Geometry check sheet. Reference: the model listing, model coordinates, mm. Round coordinates to 2 decimals unless told otherwise and drop trailing zeros. Order: outer loops, then holes, each group sorted by start corner. A loop starts at its lowest first (then second) coordinate and runs counter-clockwise, first axis right, second up.
(1) Sectioned sample at A-A (y = 2.25). Record the boundary of the cut face in (x, z), plus the area to 3 significant figures.
(2) Sectioned sample at B-B (x = 86.5). Record the boundary of the cut face in (y, z), plus the area to 3 significant figures.
(3) Material ranges on line 1 along Z through (x, y) = (93.5, 3); line 2 along X through (y, z) = (3.65, 127), recorded low to high.
Autodesk Fusion 360 part; units mm, degrees
sketch "Sketch1" plane through (0, 0, 0) normal (0, 1, 0) x (1, 0, 0)
  line L0 (0, 0) -> (170, 0)
  line L1 (170, 0) -> (170, -376)
  line L2 (170, -376) -> (0, -376)
  line L3 (0, -376) -> (0, 0)
  dimension "d1" = 170
  dimension "d2" = 376
extrude "Extrude1" add sketch "Sketch1" along normal blind 5
sketch "Sketch2" plane through (0, 0, 0) normal (-1, 0, 0) x (0, 0, 1)
  line L0 (0, 0) -> (376, 0)
  line L1 (376, 0) -> (376, 5)
  line L2 (376, 5) -> (0, 5)
  line L3 (0, 5) -> (0, 0)
extrude "Extrude2" cut 1 faces at (56.6667, 1.6667, 0) along direction (0, 0, 1) blind 3
extrude "Extrude3" cut 1 faces at (170, 1.6667, 127.3333) along direction (-1, 0, 0) blind 3
extrude "Extrude4" add 1 faces at (55.6667, 1.6667, 3) along direction (0, 0, -1) blind 3
extrude "Extrude5" add 1 faces at (167, 1.6667, 250.6667) along direction (1, 0, 0) blind 2
extrude "Extrude6" add 1 faces at (56.3333, 1.6667, 376) along direction (0, 0, 1) blind 2
extrude "Extrude7" add 1 faces at (169, 3.3333, 252) along direction (1, 0, 0) blind 3
sketch "Sketch3" plane through (0, 5, 0) normal (0, 1, 0) x (-1, 0, 0)
  line L0 (-172, 0) -> (0, 0)
  line L1 (0, 0) -> (0, 378)
  line L2 (0, 378) -> (-172, 378)
  line L3 (-172, 378) -> (-172, 0)
  line L4 (-61, 248) -> (-111, 248)
  line L5 (-111, 248) -> (-111, 278)
  line L6 (-111, 278) -> (-61, 278)
  line L7 (-61, 278) -> (-61, 248)
  line L8 (-61, 100) -> (-111, 100)
  line L9 (-111, 100) -> (-111, 130)
  line L10 (-111, 130) -> (-61, 130)
  line L11 (-61, 130) -> (-61, 100)
  dimension "d17" = 50
  dimension "d18" = 30
  dimension "d19" = 50
  dimension "d20" = 30
  dimension "d21" = 100
  dimension "d22" = 100
  dimension "d23" = 61
  dimension "d24" = 61
extrude "Extrude8" cut sketch "Sketch3" against normal blind 5 contours L4 L5 L6 L7 | L8 L9 L10 L11
Answer below:
1. outline: (0, 0) - (172, 0) - (172, 378) - (0, 378) - close; hole (61, 100) - (111, 100) - (111, 130) - (61, 130) - close; hole (61, 248) - (111, 248) - (111, 278) - (61, 278) - close
1. area: 62,000 mm2
2. outline: (0, 0) - (5, 0) - (5, 100) - (0, 100) - close; (0, 130) - (5, 130) - (5, 248) - (0, 248) - close; (0, 278) - (5, 278) - (5, 378) - (0, 378) - close
2. area: 1,590 mm2
3. line 1: z = 0 to 100, 130 to 248, 278 to 378
3. line 2: x = 0 to 61, 111 to 172
